For this review, take the finished solid that the model builds, in its own axes (mm). Face numbers are marked on the shaded views. A direction names the side the tool comes from. Coordinates: 2 decimals unless noted, no trailing zeros. Order: outer loops, then holes, each group sorted by start corner. A loop starts at its lowest first (then second) coordinate and runs counter-clockwise, first axis right, second up. Notation, with made-up numbers: (6.25, 2.25) - (64.25, 2.25) arc R5 cw to (64.25, 10.25) - close; hole circle Ø4 at (-23.75, -29.5). An arc over 180 degrees is marked (long way). One line per item, written item: value. Start each with the question number.
(1) Clearance check with flat-ended pins moving along their axes: pin 1 (8.5 mm diameter, centred on x = 4.5, y = 35, fed in from +Z); pin 2 (3 mm diameter, centred on x = 15, z = 10.5, fed in from -Y); pin 3 (6.5 mm diameter, centred on y = 14, z = 9, fed in from -X). State where each tip first meets the part, or that it passes through.
(2) Consider section A-A on x = 32.5. Write out the cut boundary in (y, z).
(3) For the marked faces 1, 2, 3, 4 and 5, list the 3-axis set-ups (+Z, -Z, +X, -X, +Y, -Y) from which the entire face can be reached by the end or side of a thin tool; tool diameter is ignored.
(4) Mouldability with a two-part tool opening along X and no side actions: class the marked faces 6, 7, 8 and 9 as released by +X, released by -X, zero draft, split by the parting line, or undercut.
(5) To check wall thickness, follow line 1 along Y through (x, z) = (3.5, 0.65); line 2 along X through (y, z) = (33.5, 1.6). State the ranges of each line that lie inside material, in increasing order.
(6) Consider section C-C on z = 7. Write out the cut boundary in (x, y), then the cut area to 3 significant figures.
```python
from build123d import *

# Parameters (mm, degrees)
F0_R     = 2
F1_DEPTH = 6.5
F3_DEPTH = 4
F4_R     = 4
F5_DEPTH = 6
F6_SIZE  = 1.99999


# Not quite as in the source:
# - a fillet or chamfer is up to 0.001 mm smaller than in the source, because OpenCascade refuses the exact size


with BuildPart() as f1:
    # F0 (on Top) → F1 (new body)
    with BuildSketch(Plane.XY):
        with BuildLine():
            Line((37, 7), (7, 37))
            ThreePointArc((7, 37), (0, 37), (0, 30))
            Line((0, 30), (30, 0))
            ThreePointArc((30, 0), (37, 0), (37, 7))
        make_face()
        with Locations((33.5, 3.5)):
            Circle(F0_R, mode=Mode.SUBTRACT)
        with Locations((3.5, 33.5)):
            Circle(F0_R, mode=Mode.SUBTRACT)
    extrude(amount=F1_DEPTH)

    # F2 (on face) → F3 (cut)
    with BuildSketch(Plane.XY.offset(6.5)):
        with BuildLine():
            Line((10.5, 33.5), (7, 37))
            ThreePointArc((7, 37), (0, 37), (0, 30))
            Line((0, 30), (3.5, 26.5))
            Line((3.5, 26.5), (10.5, 33.5))
        make_face()
        with BuildLine():
            Line((26.5, 3.5), (30, 0))
            ThreePointArc((30, 0), (37, 0), (37, 7))
            Line((37, 7), (33.5, 10.5))
            Line((33.5, 10.5), (26.5, 3.5))
        make_face()
    extrude(amount=-F3_DEPTH, mode=Mode.SUBTRACT)

    # F4 (on face) → F5 (join)
    with BuildSketch(Plane.XY.offset(6.5)):
        with BuildLine():
            ThreePointArc((3.5, 6.9), (5.904163056, 5.904163056), (6.9, 3.5))
            Line((6.9, 3.5), (6.9, 0.1))
            Line((6.9, 0.1), (23.1, 0.1))
            Line((23.1, 0.1), (33.5, 10.5))
            Line((33.5, 10.5), (10.5, 33.5))
            Line((10.5, 33.5), (0.1, 23.1))
            Line((0.1, 23.1), (0.1, 6.9))
            Line((0.1, 6.9), (3.5, 6.9))
        make_face()
        with Locations((9.8639610307, 9.8639610307)):
            Circle(F4_R, mode=Mode.SUBTRACT)
    extrude(amount=F5_DEPTH)

    # F6 (size 2 in the source; OpenCascade refuses exactly that, so slightly less here)
    f6_edges = [f1.edges().sort_by_distance(p)[0] for p in [
        (7, 30, 2.5),
        (15, 15, 6.5),
        (30, 7, 2.5),
    ]]
    chamfer(f6_edges, length=F6_SIZE)


solid = f1.part
```
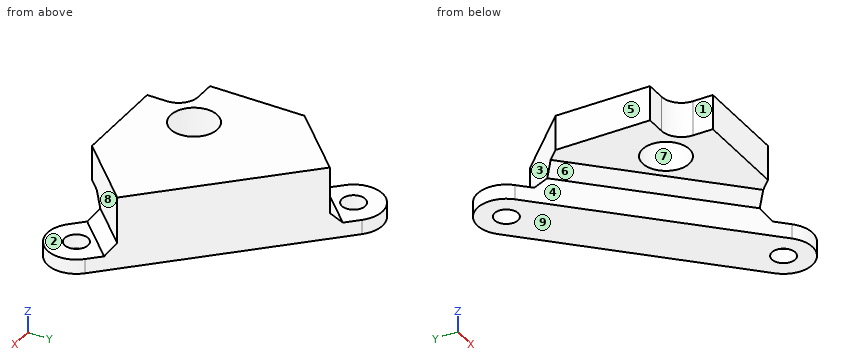
Geometry check:
1. pin 1: stops at z = 3.45
1. pin 2: stops at y = 0.1
1. pin 3: stops at x = 0.1
2. outline: (-1.35, 0) - (1.77, 0) - (1.77, 2.5) - (-1.35, 2.5) - close; (5.23, 0) - (11.5, 0) - (11.5, 12.5) - (9.5, 12.5) - (9.5, 4.5) - (6.67, 2.5) - (5.23, 2.5) - close
3. face 1: +Z, -Z, -X, -Y
3. face 2: +Z, +X, -Y
3. face 3: +Z, -X, +Y
3. face 4: -Z, -X, -Y
3. face 5: +Z, -Z, -X, +Y, -Y
4. face 6: released by -X
4. face 7: undercut
4. face 8: released by +X
4. face 9: zero draft
5. line 1: y = 26.5 to 31.5, 35.5 to 38.45
5. line 2: x = -1.45 to 1.5, 5.5 to 10.5
6. outline: (0.1, 6.9) - (3.5, 6.9) arc R3.4 cw to (6.9, 3.5) - (6.9, 0.1) - (23.1, 0.1) - (33.5, 10.5) - (10.5, 33.5) - (0.1, 23.1) - close; hole circle Ø8 at (9.86, 9.86)
6. area: 649 mm^2
